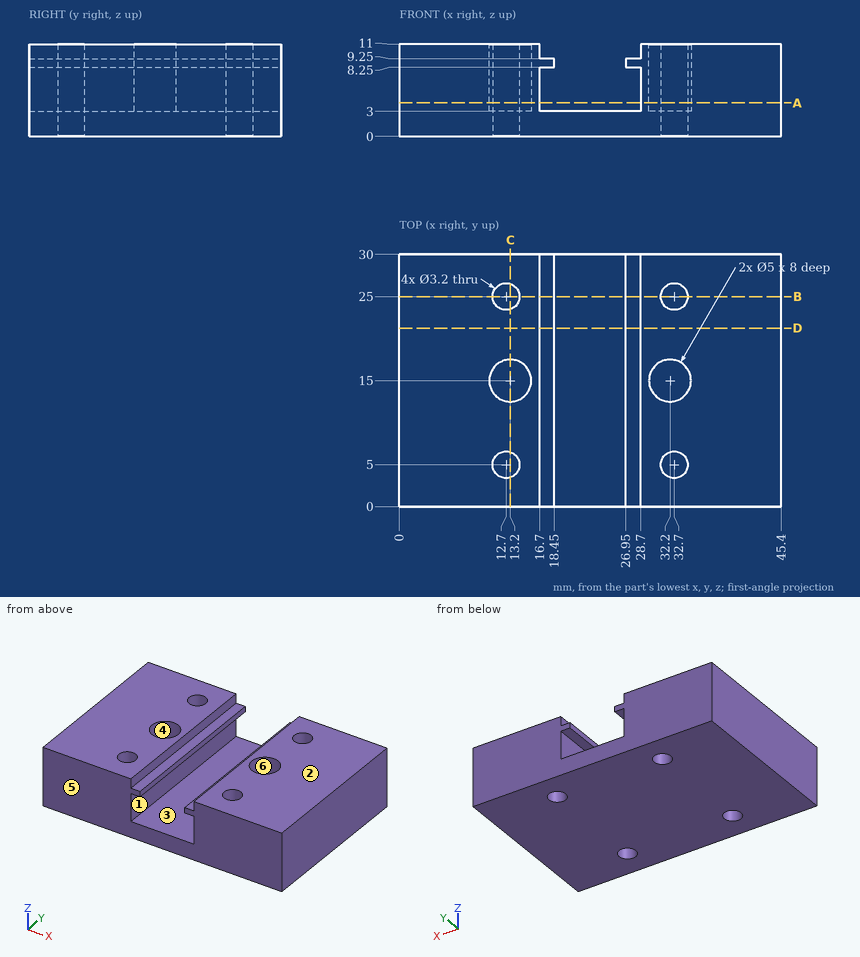
Geometry: see drawing. Coordinates: mm, zero at the bounding-box minimum. A direction names the side the tool comes from. Coordinates: 2 decimals unless noted, no trailing zeros. Order: outer loops, then holes, each group sorted by start corner. A loop starts at its lowest first (then second) coordinate and runs counter-clockwise, first axis right, second up. Notation, with made-up numbers: M -31.5,60 L 12.5,60 A24 ccw 12.5,70 Z; hole C 20.25,75.25 d5. An arc over 180 degrees is marked long. Write item = value, one per line. Start each with the question number.
(1) First-contact query: P1, Ø4, axis at x = 23, y = 9.5, coming from the +Z side; P2, Ø0.9, axis at x = 28, y = 19.5, coming from the +Z side. Flat tips, straight axial feed; report the tip coordinate or a pass-through.
(2) Section D-D on y = 21.25. Output: boundary loops of the cut face in (x, z).
(3) Reachability of the marked faces 1 and 2 from +Z, -Z, +X, -X, +Y, -Y: full face, straight path, thin tool, end or side. Return the list, or none.
(4) Section C-C on x = 13.2. Output: boundary loops of the cut face in (y, z), and give its area (3 significant figures).
(5) Line query: line 1 along X through (y, z) = (29, 5.25); line 2 along Y through (x, z) = (32.7, 5.25); line 3 along X through (y, z) = (6, 6.25). Output: solid intervals per line, ascending. Write a range as [from, to].
(6) Pull-direction query (Y, two-part tool) for the marked faces 3, 4, 5 and 6; classes: released by +Y, released by -Y, zero draft, split by the parting line, or undercut.
(7) Section B-B on y = 25. Output: boundary loops of the cut face in (x, z).
(8) Section A-A on z = 4. Output: boundary loops of the cut face in (x, y), and give its area (3 significant figures).
Result set:
q1.P1 = 3
q1.P2 = 9.25
q2.outline = M 0,0 L 45.4,0 L 45.4,11 L 28.7,11 L 28.7,9.25 L 26.95,9.25 L 26.95,8.25 L 28.7,8.25 L 28.7,3 L 16.7,3 L 16.7,8.25 L 18.45,8.25 L 18.45,9.25 L 16.7,9.25 L 16.7,11 L 0,11 Z
q3.face_1 = +Y, -Y
q3.face_2 = +Z, +X, -X, +Y, -Y
q4.outline = M 0,0 L 3.48,0 L 3.48,11 L 0,11 Z; M 6.52,0 L 23.48,0 L 23.48,11 L 17.5,11 L 17.5,3 L 12.5,3 L 12.5,11 L 6.52,11 Z; M 26.52,0 L 30,0 L 30,11 L 26.52,11 Z
q4.area = 223 mm²
q5.line_1 = [0, 16.7], [28.7, 45.4]
q5.line_2 = [0, 3.4], [6.6, 12.55], [17.45, 23.4], [26.6, 30]
q5.line_3 = [0, 11.45], [13.95, 16.7], [28.7, 31.45], [33.95, 45.4]
q6.face_3 = zero draft
q6.face_4 = undercut
q6.face_5 = released by -Y
q6.face_6 = undercut
q7.outline = M 0,0 L 11.1,0 L 11.1,11 L 0,11 Z; M 14.3,0 L 31.1,0 L 31.1,11 L 28.7,11 L 28.7,9.25 L 26.95,9.25 L 26.95,8.25 L 28.7,8.25 L 28.7,3 L 16.7,3 L 16.7,8.25 L 18.45,8.25 L 18.45,9.25 L 16.7,9.25 L 16.7,11 L 14.3,11 Z; M 34.3,0 L 45.4,0 L 45.4,11 L 34.3,11 Z
q8.outline = M 0,0 L 16.7,0 L 16.7,30 L 0,30 Z; M 28.7,0 L 45.4,0 L 45.4,30 L 28.7,30 Z; hole C 13.2,15 d5; hole C 12.7,5 d3.2; hole C 12.7,25 d3.2; hole C 32.2,15 d5; hole C 32.7,5 d3.2; hole C 32.7,25 d3.2
q8.area = 931 mm²
